The model under review builds one solid part; all positions refer to its coordinate system, in mm. A direction names the side the tool comes from. Coordinates: 2 decimals unless noted, no trailing zeros. Write each loop counter-clockwise with the first axis right and the second up, starting at its lowest first coordinate (ties: lowest second). Pieces come first, ordered by that corner, then holes.
```python
from build123d import *

# Parameters (mm, degrees)
SKETCH1_W           = 18
SKETCH1_H           = 105.4
BOSS_EXTRUDE1_DEPTH = 3
SKETCH3_W           = 3
SKETCH3_H           = 41.865
CUT_EXTRUDE2_DEPTH  = 3
SKETCH5_W           = 3
SKETCH5_H           = 18.88
SKETCH5_H_2         = 33.86
SKETCH5_H_3         = 18.78
CUT_EXTRUDE5_DEPTH  = 3


with BuildPart() as part:
    # Sketch1 → Boss-Extrude1 (new body)
    with BuildSketch(Plane(origin=(0, 0, 0), x_dir=(0, 0, -1), z_dir=(1, 0, 0))):
        Rectangle(SKETCH1_W, SKETCH1_H)
    extrude(amount=BOSS_EXTRUDE1_DEPTH)

    # Sketch3 → Cut-Extrude2 (cut)
    with BuildSketch(Plane(origin=(3, 0, 0), x_dir=(0, 0, -1), z_dir=(1, 0, 0))):
        with Locations((7.5, -31.7675)):
            Rectangle(SKETCH3_W, SKETCH3_H)
        with Locations((7.5, 31.7675)):
            Rectangle(SKETCH3_W, SKETCH3_H)
    extrude(amount=-CUT_EXTRUDE2_DEPTH, mode=Mode.SUBTRACT)

    # Sketch5 → Cut-Extrude5 (cut)
    with BuildSketch(Plane.ZY):
        with Locations((7.5, -43.26)):
            Rectangle(SKETCH5_W, SKETCH5_H)
        with Locations((7.5, 0.04)):
            Rectangle(SKETCH5_W, SKETCH5_H_2)
        with Locations((7.5, 43.31)):
            Rectangle(SKETCH5_W, SKETCH5_H_3)
    extrude(amount=-CUT_EXTRUDE5_DEPTH, mode=Mode.SUBTRACT)


solid = part.part
```
Item 1: Machinability: for faces 5 (the face through (2, 10.835, -7)), 6 (the face through (1, -43, 6)), 7 (the face through (2, -32, -6)), 8 (the face through (1, 43, 6)), which of the approach directions +Z, -Z, +X, -X, +Y, -Y give a long, thin tool a straight path to every point of the face, cutting with its end or side? Answer none if there is none.
Solved:
face 5: -Z, +X, -X, +Y
face 6: +Z, +X, -X, -Y
face 7: -Z, +X, -X, -Y
face 8: +Z, +X, -X, +Y
Item 2: Take a section at D-D, the plane y = -37. Write out the cut boundary in (x, z), plus the area to 3 significant figures.
Solved:
outline: (0, -6) - (3, -6) - (3, 6) - (0, 6) - close
area: 36.0 mm2
Item 3: For pin 1 (1.5 mm diameter, centred on x = 1, z = 7, fed in from +Y); pin 2 (10 mm diameter, centred on y = 33, z = -6.5, fed in from -X); pin 3 (1.5 mm diameter, centred on x = 1, y = -1, fed in from +Z); pin 4 (1.5 mm diameter, centred on x = 1.5, z = 7, fed in from -Y), all flat-tipped, find the tip position at first contact; note any pin that passes through.
Solved:
pin 1: stops at y = 33.92
pin 2: stops at x = 0
pin 3: stops at z = 6
pin 4: stops at y = -33.82
Item 4: Take a section at B-B, the plane x = 2.25. Write out the cut boundary in (y, z) (3 decimals), plus the area to 3 significant figures.
Solved:
outline: (-52.7, -6) - (-10.835, -6) - (-10.835, -9) - (10.835, -9) - (10.835, -6) - (52.7, -6) - (52.7, 6) - (33.92, 6) - (33.92, 9) - (16.97, 9) - (16.97, 6) - (-16.89, 6) - (-16.89, 9) - (-33.82, 9) - (-33.82, 6) - (-52.7, 6) - close
area: 1,430 mm2
Item 5: To check wall thickness, follow line 1 along Y through (x, z) = (0.5, 8); line 2 along Z through (x, y) = (0.75, 28); line 3 along Z through (x, y) = (2.5, 46.5). State the ranges of each line that lie inside material, in increasing order.
Solved:
line 1: y = -33.82 to -16.89, 16.97 to 33.92
line 2: z = -6 to 9
line 3: z = -6 to 6
Item 6: Take a section at A-A, the plane z = 7. Write out the cut boundary in (x, y), plus the area to 3 significant figures.
Solved:
outline: (0, -33.82) - (3, -33.82) - (3, -16.89) - (0, -16.89) - close; (0, 16.97) - (3, 16.97) - (3, 33.92) - (0, 33.92) - close
area: 102 mm2
Item 7: Take a section at C-C, the plane y = 30. Write out the cut boundary in (x, z).
Solved:
outline: (0, -6) - (3, -6) - (3, 9) - (0, 9) - close
Item 8: Mouldability with a two-part tool opening along Y and no side actions: class faces 1 (the face through (1, 52.7, 0)), 2 (the face through (1, -25, 9)), 3 (the face through (1, 0, 6)), 4 (the face through (1, -16.89, 7)) as pulls with the +Y half, pulls with the -Y half, needs draft (parallel to the pull), parting line crosses it, or undercut.
Solved:
face 1: pulls with the +Y half
face 2: needs draft
face 3: undercut
face 4: undercut
